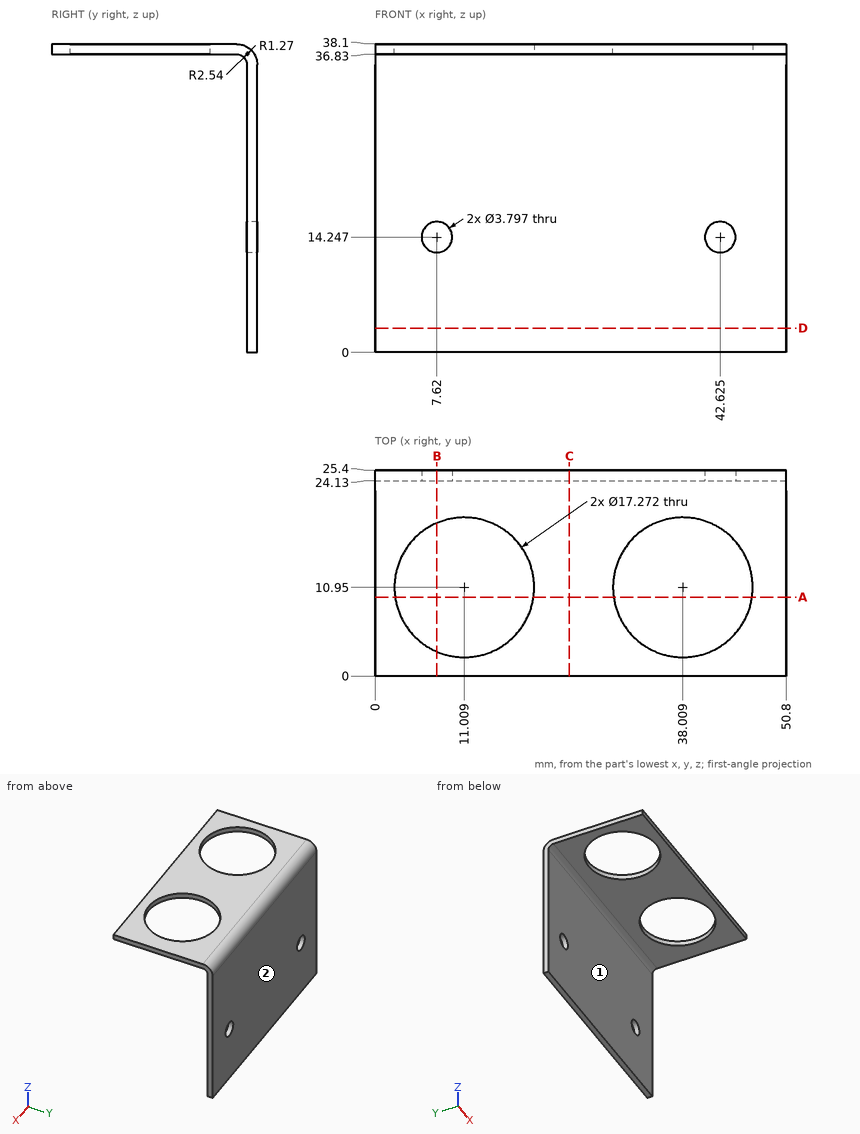
Could you check a few things on this drawing? It's one solid part, dimensions in mm from its lowest x, y, z. A direction names the side the tool comes from. Coordinates: 2 decimals unless noted, no trailing zeros. Write each loop counter-clockwise with the first axis right and the second up, starting at its lowest first coordinate (ties: lowest second). Pieces come first, ordered by that corner, then holes. Notation, with made-up numbers: (17.25, 41) - (58.25, 41) arc R36 ccw to (58.25, 76) - close; hole circle Ø9 at (-0.75, 59). An arc over 180 degrees is marked (long way). Return JSON: item names as keys, results as strings. Group by question number.
Item 1: Which directions (+Z, -Z, +X, -X, +Y, -Y) give clear straight access to the entire face, cutting with the end or side of a thin tool? Please do the marked faces 1 and 2.
Item 2: Please list where these lines run through material, in increasing order: probe 1 along Y at (x, z) = (32.5, 22.5); probe 2 along Z at (x, y) = (21, 6.25); probe 3 along Z at (x, y) = (32.5, 24).
Item 3: If we section it at D-D (z = 3): Write out the boundary of the cut face in (x, y).
Item 4: I'm going to push flat-ended pins straight in: pin 1 Ø4.5 at (x, z) = (7.62, 14.25) entering from -Y; pin 2 Ø1.5 at (x, y) = (5.5, 21.5) entering from -Z; pin 3 Ø5 at (x, y) = (43, 5.5) entering from +Z. Where does each tip first touch, or does it pass through?
Item 5: If we section it at A-A (y = 9.75): Write out the boundary of the cut face in (x, z).
Item 6: If we section it at B-B (x = 7.62): Write out the boundary of the cut face in (y, z).
Item 7: If we section it at C-C (x = 24): Write out the boundary of the cut face in (y, z).
Return value:
{
 "1": {"face 1": "-Z, +X, -X, -Y", "face 2": "+Z, -Z, +X, -X, +Y"},
 "2": {"probe 1": "y = 24.13 to 25.4", "probe 2": "z = 36.83 to 38.1", "probe 3": "z = 36.12 to 37.83"},
 "3": {"outline": "(0, 24.13) - (50.8, 24.13) - (50.8, 25.4) - (0, 25.4) - close"},
 "4": {"pin 1": "stops at y = 24.13", "pin 2": "stops at z = 36.83", "pin 3": "stops at z = 38.1"},
 "5": {"outline": "(0, 36.83) - (2.46, 36.83) - (2.46, 38.1) - (0, 38.1) - close; (19.56, 36.83) - (29.46, 36.83) - (29.46, 38.1) - (19.56, 38.1) - close; (46.56, 36.83) - (50.8, 36.83) - (50.8, 38.1) - (46.56, 38.1) - close"},
 "6": {"outline": "(0, 36.83) - (3.01, 36.83) - (3.01, 38.1) - (0, 38.1) - close; (18.89, 36.83) - (22.86, 36.83) arc R1.27 cw to (24.13, 35.56) - (24.13, 16.15) - (25.4, 16.15) - (25.4, 35.56) arc R2.54 ccw to (22.86, 38.1) - (18.89, 38.1) - close; (24.13, 0) - (25.4, 0) - (25.4, 12.35) - (24.13, 12.35) - close"},
 "7": {"outline": "(0, 36.83) - (22.86, 36.83) arc R1.27 cw to (24.13, 35.56) - (24.13, 0) - (25.4, 0) - (25.4, 35.56) arc R2.54 ccw to (22.86, 38.1) - (0, 38.1) - close"}
}
